```python
from build123d import *

# Parameters (mm, degrees)
SKETCH1_R               = 19.05
BOSS_EXTRUDE1_DEPTH     = 3.175
SKETCH2_R               = 9.525
BOSS_EXTRUDE2_DEPTH     = 57.15
SKETCH3_R               = 19.05
BOSS_EXTRUDE3_DEPTH     = 3.175
SKETCH4_R               = 3.81
CUT_EXTRUDE1_DEPTH      = 63.5
CUT_EXTRUDE2_REACH      = 30.575
CUT_EXTRUDE2_END_RADIUS = 3.81
SKETCH5_R               = 1.5
SKETCH6_R               = 1.5875
CUT_EXTRUDE3_DEPTH      = 20.05
CUT_EXTRUDE3_DEPTH_BACK = 20.05


with BuildPart() as part:
    # Sketch1 → Boss-Extrude1 (new body)
    with BuildSketch(Plane(origin=(0, 0, 0), x_dir=(0, 0, -1), z_dir=(1, 0, 0))):
        Circle(SKETCH1_R)
    extrude(amount=BOSS_EXTRUDE1_DEPTH)

    # Sketch2 → Boss-Extrude2 (add)
    with BuildSketch(Plane(origin=(3.175, 0, 0), x_dir=(0, 0, -1), z_dir=(1, 0, 0))):
        Circle(SKETCH2_R)
    extrude(amount=BOSS_EXTRUDE2_DEPTH)

    # Sketch3 → Boss-Extrude3 (add)
    with BuildSketch(Plane(origin=(60.325, 0, 0), x_dir=(0, 0, -1), z_dir=(1, 0, 0))):
        Circle(SKETCH3_R)
    extrude(amount=BOSS_EXTRUDE3_DEPTH)

    # Sketch4 → Cut-Extrude1 (cut)
    with BuildSketch(Plane(origin=(63.5, 0, 0), x_dir=(0, 0, -1), z_dir=(1, 0, 0))):
        Circle(SKETCH4_R)
    extrude(amount=-CUT_EXTRUDE1_DEPTH, mode=Mode.SUBTRACT)

    # Cut-Extrude2: up to this cylinder (the profile starts outside it)
    cut_extrude2_end = Plane(origin=(8.630484, 0, 0), z_dir=(1, 0, 0)) * Cylinder(CUT_EXTRUDE2_END_RADIUS, 69.77, mode=Mode.PRIVATE)
    # Sketch5 → Cut-Extrude2 (cut, up to the surface)
    with BuildSketch(Plane(origin=(0, 0, -9.525), x_dir=(-1, 0, 0), z_dir=(0, 0, -1)), mode=Mode.PRIVATE) as cut_extrude2_sk1:
        with Locations((-8.630483707, 0)):
            Circle(SKETCH5_R)
    cut_extrude2_tool1 = extrude(cut_extrude2_sk1.sketch, amount=-CUT_EXTRUDE2_REACH, mode=Mode.PRIVATE) - cut_extrude2_end
    add(cut_extrude2_tool1.solids().sort_by_distance((8.630484, 0, -9.525))[0], mode=Mode.SUBTRACT)

    # Sketch6 → Cut-Extrude3 (cut, two sides)
    with BuildSketch(Plane(origin=(0, 0, 0), x_dir=(1, 0, 0), z_dir=(0, 1, 0))) as cut_extrude3_sk:
        with Locations(Location((32.798989334, 0, 0), (0, 0, 270))):  # turned: the seam where the file's is
            Circle(SKETCH6_R)
    extrude(amount=CUT_EXTRUDE3_DEPTH, mode=Mode.SUBTRACT)
    extrude(cut_extrude3_sk.sketch, amount=-CUT_EXTRUDE3_DEPTH_BACK, mode=Mode.SUBTRACT)


solid = part.part
```
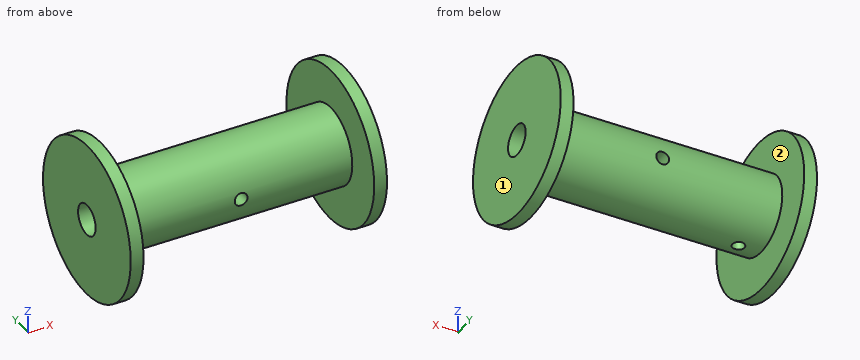
Part model, mm, in its own coordinate system. Face numbers are marked on the shaded views. A direction names the side the tool comes from. Round coordinates to 2 decimals unless told otherwise and drop trailing zeros. Write each loop counter-clockwise with the first axis right and the second up, starting at its lowest first coordinate (ties: lowest second). Pieces come first, ordered by that corner, then holes. Notation, with made-up numbers: M 82,18 L 123,18 A18 cw 123,44 Z; hole C 35,37 d6. An arc over 180 degrees is marked long. Answer as CSV lines item,"result". Start each with the question number.
1) Drop flat-ended pins along their axis: pin 1 (3.5 mm diameter, centred on x = 32.8, z = 0, fed in from +Y) (3 decimals); pin 2 (1 mm diameter, centred on x = 54, y = -2, fed in from -Z); pin 3 (1.9 mm diameter, centred on x = 32.8, z = 0, fed in from +Y); pin 4 (2 mm diameter, centred on x = 53.5, y = -9, fed in from +Z). Give the stop position or say it passes through.
2) Band-saw the part on C-C (y = -13.5). List the corners of the cut face in (x, z) (3 decimals).
3) Drill centre lines: L1, parallel to X at y = 0, z = -5.5; L2, parallel to X at y = -5, z = 17 (3 decimals); L3, parallel to Y at x = 33.5, z = -3.5. Where is each one in solid material? Low to high.
4) Which spindle directions (+Z, -Z, +X, -X, +Y, -Y) get a long thin tool onto all of the face, cutting with end or side? Do the marked faces 1 and 2. Say none if no direction does.
5) Band-saw the part on A-A (z = 0). List the corners of the cut face in (x, y) (3 decimals), then the cut area to 3 significant figures.
6) Band-saw the part on B-B (y = 0). List the corners of the cut face in (x, z) (3 decimals), then the cut area to 3 significant figures.
7) Band-saw the part on D-D (x = 16). List the corners of the cut face in (y, z) (3 decimals), then the cut area to 3 significant figures.
Worked out:
1,pin 1,"y = 9.525"
1,pin 2,"z = -9.41"
1,pin 3,"through"
1,pin 4,"z = 5.17"
2,outline,"M 0,-13.441 L 3.175,-13.441 L 3.175,13.441 L 0,13.441 Z; M 60.325,-13.441 L 63.5,-13.441 L 63.5,13.441 L 60.325,13.441 Z"
3,L1,"0 to 7.13, 10.13 to 63.5"
3,L2,"0 to 3.175, 60.325 to 63.5"
3,L3,"-8.86 to -1.51, 1.51 to 8.86"
4,face 1,"+Z, -Z, +X, +Y, -Y"
4,face 2,"none"
5,outline,"M 0,-19.05 L 3.175,-19.05 L 3.175,-9.525 L 31.211,-9.525 L 31.211,-3.81 L 0,-3.81 Z; M 0,3.81 L 31.211,3.81 L 31.211,9.525 L 3.175,9.525 L 3.175,19.05 L 0,19.05 Z; M 34.386,-9.525 L 60.325,-9.525 L 60.325,-19.05 L 63.5,-19.05 L 63.5,-3.81 L 34.386,-3.81 Z; M 34.386,3.81 L 63.5,3.81 L 63.5,19.05 L 60.325,19.05 L 60.325,9.525 L 34.386,9.525 Z"
5,area,"810 mm²"
6,outline,"M 0,-19.05 L 3.175,-19.05 L 3.175,-9.525 L 7.13,-9.525 L 7.13,-3.81 L 0,-3.81 Z; M 0,3.81 L 63.5,3.81 L 63.5,19.05 L 60.325,19.05 L 60.325,9.525 L 3.175,9.525 L 3.175,19.05 L 0,19.05 Z; M 10.13,-9.525 L 60.325,-9.525 L 60.325,-19.05 L 63.5,-19.05 L 63.5,-3.81 L 10.13,-3.81 Z"
6,area,"830 mm²"
7,outline,"C 0,0 d19.05; hole C 0,0 d7.62"
7,area,"239 mm²"
